Check sheet for the modelled part. Datum: model origin and axes. Units: mm. A direction names the side the tool comes from. Give positions to 0.01 mm unless a question says otherwise; leave off trailing zeros. Write each loop counter-clockwise with the first axis right and the second up, starting at its lowest first coordinate (ties: lowest second). Pieces come first, ordered by that corner, then holes. Notation, with made-up numbers: (-23, 10) -> (11, 10) arc R21 ccw to (11, 24) -> close; hole circle Ø11 at (12.5, -18.75). An arc over 180 degrees is marked (long way). Answer as a JSON object with one key per item and string values.
Autodesk Fusion 360 part; units mm, degrees
sketch "Schizzo1" plane through (0, 0, 0) normal (0, 0, 1) x (1, 0, 0)
  line L0 (64.6508, 75.5456) -> (160.3508, 75.5456) construction
  line L1 (160.3508, 75.5456) -> (160.3508, 23.8456) construction
  line L2 (160.3508, 23.8456) -> (64.6508, 23.8456) construction
  line L3 (64.6508, 23.8456) -> (64.6508, 75.5456) construction
  line L4 (64.6508, 49.6956) -> (160.3508, 49.6956) construction
  line L5 (112.5008, 75.5456) -> (112.5008, 23.8456) construction
  line L6 (160.2508, 23.9456) -> (64.7508, 23.9456)
  line L7 (64.7508, 23.9456) -> (64.7508, 75.4456)
  line L8 (64.7508, 75.4456) -> (160.2508, 75.4456)
  line L9 (160.2508, 75.4456) -> (160.2508, 23.9456)
  line L10 (160.2508, 23.9456) -> (64.7508, 75.4456) construction
  line L11 (64.7508, 23.9456) -> (160.2508, 75.4456) construction
  line L12 (146.3653, 67.9576) -> (78.6363, 31.4336) construction
  line L13 (78.6363, 67.9576) -> (146.3653, 31.4336) construction
  point P0 (112.5008, 49.6956)
  point P1 (112.5008, 49.6956)
  dimension "d1" = 95.7
  dimension "d2" = 51.7
  dimension "d3" = 0.1
  dimension "d4" = 0.1
extrude "Estrusione1" add sketch "Schizzo1" along normal blind 4
fillet "Raccordo1" radius 2 4 edges at (64.7508, 23.9456, 2) (64.7508, 75.4456, 2) (160.2508, 23.9456, 2) (160.2508, 75.4456, 2)
sketch "Schizzo2" plane through (0, 0, 4) normal (0, 0, 1) x (-1, 0, 0)
  arc A0 (-160.2508, -73.4456) -> (-158.2508, -75.4456) centre (-158.2508, -73.4456) ccw
  line L0 (-158.2508, -75.4456) -> (-66.7508, -75.4456)
  arc A1 (-66.7508, -75.4456) -> (-64.7508, -73.4456) centre (-66.7508, -73.4456) ccw
  line L1 (-64.7508, -73.4456) -> (-64.7508, -25.9456)
  arc A2 (-64.7508, -25.9456) -> (-66.7508, -23.9456) centre (-66.7508, -25.9456) ccw
  line L2 (-66.7508, -23.9456) -> (-158.2508, -23.9456)
  arc A3 (-158.2508, -23.9456) -> (-160.2508, -25.9456) centre (-158.2508, -25.9456) ccw
  line L3 (-160.2508, -25.9456) -> (-160.2508, -73.4456)
  line L4 (-64.7508, -75.4456) -> (-160.2508, -75.4456) construction
  line L5 (-160.2508, -75.4456) -> (-160.2508, -23.9456) construction
  line L6 (-160.2508, -23.9456) -> (-64.7508, -23.9456) construction
  line L7 (-64.7508, -23.9456) -> (-64.7508, -75.4456) construction
  line L8 (-64.7508, -49.6956) -> (-160.2508, -49.6956) construction
  line L9 (-112.5008, -75.4456) -> (-112.5008, -23.9456) construction
  line L10 (-158.2508, -73.4456) -> (-66.7508, -73.4456)
  line L11 (-66.7508, -73.4456) -> (-66.7508, -25.9456)
  line L12 (-66.7508, -25.9456) -> (-158.2508, -25.9456)
  line L13 (-158.2508, -25.9456) -> (-158.2508, -73.4456)
  line L14 (-158.2508, -73.4456) -> (-66.7508, -25.9456) construction
  line L15 (-66.7508, -73.4456) -> (-158.2508, -25.9456) construction
  line L16 (-116.0008, -25.9456) -> (-109.0008, -25.9456)
  line L17 (-109.0008, -25.9456) -> (-109.0008, -73.4456)
  line L18 (-109.0008, -73.4456) -> (-116.0008, -73.4456)
  line L19 (-116.0008, -73.4456) -> (-116.0008, -25.9456)
  line L20 (-116.0008, -25.9456) -> (-109.0008, -73.4456) construction
  line L21 (-109.0008, -25.9456) -> (-116.0008, -73.4456) construction
  line L22 (-84.5008, -72.4456) -> (-73.5008, -72.4456)
  line L23 (-73.5008, -72.4456) -> (-73.5008, -75.4456)
  line L24 (-73.5008, -75.4456) -> (-84.5008, -75.4456)
  line L25 (-84.5008, -75.4456) -> (-84.5008, -72.4456)
  line L26 (-84.5008, -72.4456) -> (-73.5008, -75.4456) construction
  line L27 (-73.5008, -72.4456) -> (-84.5008, -75.4456) construction
  line L28 (-151.5008, -72.4456) -> (-151.5008, -75.4456)
  line L29 (-151.5008, -75.4456) -> (-140.5008, -75.4456)
  line L30 (-140.5008, -72.4456) -> (-151.5008, -72.4456)
  line L31 (-140.5008, -75.4456) -> (-140.5008, -72.4456)
  line L32 (-151.5008, -72.4456) -> (-140.5008, -75.4456) construction
  line L33 (-140.5008, -72.4456) -> (-151.5008, -75.4456) construction
  line L34 (-66.7508, -73.4456) -> (-94.7508, -73.4456)
  line L35 (-94.7508, -73.4456) -> (-94.7508, -63.4456)
  line L36 (-94.7508, -63.4456) -> (-66.7508, -63.4456)
  line L37 (-66.7508, -63.4456) -> (-66.7508, -73.4456)
  line L38 (-115.7508, -73.4456) -> (-143.7508, -73.4456)
  line L39 (-143.7508, -73.4456) -> (-143.7508, -63.4456)
  line L40 (-143.7508, -63.4456) -> (-115.7508, -63.4456)
  line L41 (-115.7508, -63.4456) -> (-115.7508, -73.4456)
  line L42 (-84.5008, -26.9456) -> (-73.5008, -26.9456)
  line L43 (-73.5008, -26.9456) -> (-73.5008, -23.9456)
  line L44 (-73.5008, -23.9456) -> (-84.5008, -23.9456)
  line L45 (-84.5008, -23.9456) -> (-84.5008, -26.9456)
  line L46 (-140.5008, -26.9456) -> (-151.5008, -26.9456)
  line L47 (-140.5008, -23.9456) -> (-140.5008, -26.9456)
  line L48 (-151.5008, -26.9456) -> (-151.5008, -23.9456)
  line L49 (-151.5008, -23.9456) -> (-140.5008, -23.9456)
  point P0 (-112.5008, -49.6956)
  point P1 (-112.5008, -49.6956)
  point P2 (-79.0008, -73.9456)
  point P3 (-146.0008, -73.9456)
  dimension "d9" = 2
  dimension "d10" = 2
  dimension "d11" = 7
  dimension "d14" = 11
  dimension "d15" = 3
  dimension "d16" = 67
  dimension "d19" = 28
  dimension "d20" = 10
  dimension "d21" = 28
  dimension "d22" = 10
  dimension "d23" = 49
extrude "Estrusione2" cut sketch "Schizzo2" against normal blind 3 contours L10 L28 L30 L39 | L10 L12 L13 L19 L28 L30 L39 L40 L46 L47 L48 | L10 L19 L30 L31 L38 L39 L40 | L10 L30 L31 L38 L39 | L12 L46 L47 L48 | L10 L22 L23 L25 L34 | L10 L11 L22 L23 L25 L34 L35 L36 L37 | L10 L11 L12 L17 L35 L36 L42 L43 L45 | L12 L42 L43 L45
extrude "Estrusione4" cut sketch "Schizzo2" against normal blind 4 contours L10 L19 L30 L31 L38 L39 L40 | L10 L30 L31 L38 L39 | L10 L22 L23 L25 L34 | L10 L11 L22 L23 L25 L34 L35 L36 L37
extrude "Estrusione5" cut sketch "Schizzo2" against normal blind 2 contours L0 L10 L28 L29 L31 L38 | L2 L12 L47 L48 L49 | L0 L10 L23 L24 L25 L34 | L2 L12 L43 L44 L45
ref_plane "Piano di lavoro1" through (112.5008, 49.6956, 4) normal (0, -1, 0) x (1, 0, 0)
sketch "Schizzo3" plane through (0, 49.6956, 0) normal (0, -1, 0) x (-1, 0, 0)
  line L0 (-64.7508, -4) -> (-160.3508, -4) construction
  line L1 (-160.3508, -4) -> (-160.3508, 0) construction
  line L2 (-160.3508, 0) -> (-64.7508, 0) construction
  line L3 (-64.7508, 0) -> (-64.7508, -4) construction
  line L4 (-109.0008, -1) -> (-109.0008, -4) construction
  line L5 (-64.7508, -1) -> (-160.3508, -1) construction
  line L6 (-94.7508, -1) -> (-109.0008, -1) construction
  line L7 (-109.0008, -4) -> (-109.0008, 0) construction
  line L8 (-116, -4) -> (-116, 0) construction
  line L9 (-109.0008, -1) -> (-109.0008, -4)
  line L10 (-109.0008, -4) -> (-110.7329, -1)
  line L11 (-110.7329, -1) -> (-109.0008, -1)
  line L12 (-110.7329, -1) -> (-109.0008, -4)
  line L13 (-109.0008, -4) -> (-109.0008, -1)
  line L14 (-112.5508, -4) -> (-112.5508, 0) construction
  line L15 (-116.1008, -4) -> (-114.3688, -1)
  line L16 (-116.1008, -4) -> (-116.1008, 0) construction
  line L17 (-114.3688, -1) -> (-116.1008, -1)
  line L18 (-116.1008, -4) -> (-116.1008, -1)
  point P0 (-64.7508, -4)
  point P1 (-160.3508, 0)
  point P2 (-109.0008, -4)
  dimension "d29" = 30
extrude "Estrusione6" cut sketch "Schizzo3" along normal mid plane 40
equation "d21 = d19"
equation "d22 = d20"
1. Sectioned sample at D-D, the plane x = 106. Enter the section's corners in (y, z), plus the area to 3 significant figures.
Determined:
{"outline": "(23.95, 0) -> (75.45, 0) -> (75.45, 4) -> (73.45, 4) -> (73.45, 1) -> (25.95, 1) -> (25.95, 4) -> (23.95, 4) -> close", "area": "63.5 mm^2"}
2. Sectioned sample at B-B, the plane y = 65.5. Enter the section's corners in (x, z).
Determined:
{"outline": "(64.75, 0) -> (66.75, 0) -> (66.75, 4) -> (64.75, 4) -> close; (94.75, 0) -> (116, 0) -> (116, 1) -> (114.37, 1) -> (116, 3.83) -> (116, 4) -> (109, 4) -> (110.73, 1) -> (94.75, 1) -> close; (143.75, 0) -> (160.25, 0) -> (160.25, 4) -> (158.25, 4) -> (158.25, 1) -> (143.75, 1) -> close"}
3. Scan lines: L1, parallel to X at y = 70, z = 1.7; L2, parallel to Y at x = 106, z = 3.1; L3, parallel to X at y = 34, z = 2.65. Record each from-to range of solid material in increasing order. Write a range as [from, to].
Determined:
{"L1": "[64.75, 66.75], [109, 116], [158.25, 160.25]", "L2": "[23.95, 25.95], [73.45, 75.45]", "L3": "[64.75, 66.75], [109.78, 115.32], [158.25, 160.25]"}
4. Access from +Z, -Z, +X, -X, +Y, -Y to the whole of each face (thin tool, end or side, straight path). Record for faces 1 (the face through (115.196, 49.976, 2.433)), 2 (the face through (112, 50, 4)), 3 (the face through (140.501, 74, 3)), 4 (the face through (109.001, 72, 3)).
Determined:
{"face 1": "none", "face 2": "+Z, +X, -X, +Y, -Y", "face 3": "+Z, +Y, -Y", "face 4": "+Z"}
5. Sectioned sample at C-C, the plane y = 32.5. Enter the section's corners in (x, z).
Determined:
{"outline": "(64.75, 0) -> (160.25, 0) -> (160.25, 4) -> (158.25, 4) -> (158.25, 1) -> (114.37, 1) -> (116, 3.83) -> (116, 4) -> (109, 4) -> (110.73, 1) -> (66.75, 1) -> (66.75, 4) -> (64.75, 4) -> close"}
6. Go/stop test with flat-tipped pins: P1, Ø22, axis at x = 144, y = 50, coming from the +Z side; P2, Ø0.6, axis at y = 25, z = 3, coming from the -X side. Record where each tip stops, or that it passes through.
Determined:
{"P1": "z = 1", "P2": "x = 64.86"}
7. Mould release check, pull along Y, two halves, no side actions. Record for faces 5 (the face through (159.68, 74.844, 2.028)), 6 (the face through (132, 25.946, 3)), 7 (the face through (79, 74, 2)): released by +Y, released by -Y, zero draft, split by the parting line, or undercut.
Determined:
{"face 5": "released by +Y", "face 6": "undercut", "face 7": "zero draft"}
8. Sectioned sample at A-A, the plane x = 83. Enter the section's corners in (y, z).
Determined:
{"outline": "(23.95, 0) -> (63.45, 0) -> (63.45, 1) -> (25.95, 1) -> (25.95, 2) -> (23.95, 2) -> close; (73.45, 0) -> (75.45, 0) -> (75.45, 2) -> (73.45, 2) -> close"}
